Check sheet for the modelled part. Datum: model origin and axes. Units: mm. Face numbers are marked on the shaded views. Coordinates: 2 decimals unless noted, no trailing zeros. Loops run counter-clockwise (first coordinate to the right, second up) from the corner with the lowest first, then second, coordinate; pieces in that order, holes last. Notation, with made-up numbers: (78.5, -30) -> (85.5, -30) arc R16 ccw to (85.5, -26) -> close; hole circle Ø3 at (-26, -17). An arc over 180 degrees is marked (long way). Use CSV: the item, a comma, the result in double quotes. Start each with the question number.
1. Thickness scan on L1, parallel to Y at x = 52.1, z = -4.4; L2, parallel to Z at x = 45, y = 1.5; L3, parallel to X at y = 46, z = -2.9. Record the ranges inside material, lowest first.
2. Sectioned sample at B-B, the plane x = 47. Record the cut outline in (y, z).
3. Release check for a two-part mould opening along Y. For the marked faces 1 and 2 record: pulls with the +Y half, pulls with the -Y half, needs draft (parallel to the pull), parting line crosses it, or undercut.
4. Sectioned sample at A-A, the plane z = -0.7. Record the cut outline in (x, y), and give its area (3 significant figures).
5. Gauge pin test, flat ends, axial feed: pin 1 (3.5 mm diameter, centred on x = 52.1, y = 30.4, fed in from +Z); pin 2 (1 mm diameter, centred on x = 41, y = 32, fed in from +Z); pin 3 (2.5 mm diameter, centred on x = 0, y = 0, fed in from +Z). Record the tip position at first contact, or that the pin passes through.
6. Sectioned sample at C-C, the plane y = 23.5. Record the cut outline in (x, z), and give its area (3 significant figures).
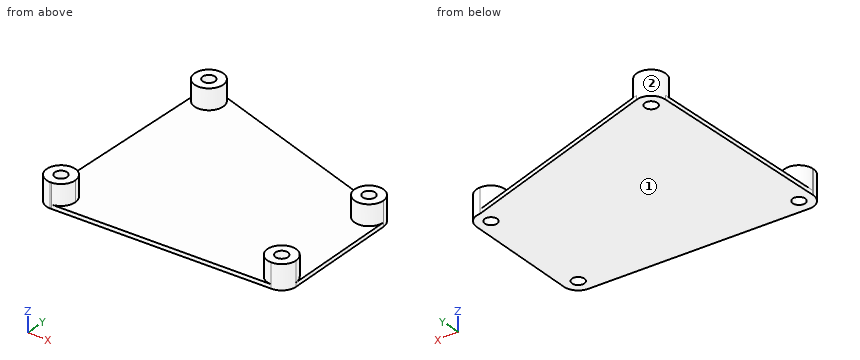
```python
from build123d import *

# Parameters (mm, degrees)
SKETCH1_R           = 3.5
SKETCH1_R_2         = 1.5
BOSS_EXTRUDE2_DEPTH = 6
CUT_EXTRUDE2_DEPTH  = 5


with BuildPart() as part:
    # Sketch1 → Boss-Extrude2 (new body)
    # profile 1 of 5: a face of its own
    with BuildSketch(Plane.XY):
        with BuildLine():
            ThreePointArc((4.8, 45.6), (1.3, 42.1), (-2.2, 45.6))
            Line((-2.2, 45.6), (-3.49431537, 0.199399342))
            ThreePointArc((-3.49431537, 0.199399342), (0.099740178, 3.498578554), (3.5, 0))
            ThreePointArc((3.5, 0), (2.590648868, -2.353409961), (0.33512089, -3.483919343))
            Line((0.33512089, -3.483919343), (52.1, -1))
            ThreePointArc((52.1, -1), (49.625126266, 4.974873734), (55.6, 2.5))
            Line((55.6, 2.5), (55.6, 30.4))
            ThreePointArc((55.6, 30.4), (49.625126266, 27.925126266), (52.1, 33.9))
            Line((52.1, 33.9), (2.312759359, 48.950271404))
            ThreePointArc((2.312759359, 48.950271404), (4.110218653, 47.686305616), (4.8, 45.6))
        make_face()
    # profile 2 of 5: a face of its own
    with BuildSketch(Plane.XY):
        with Locations((1.3, 45.6)):
            Circle(SKETCH1_R)
        with Locations((1.3, 45.6)):
            Circle(SKETCH1_R_2, mode=Mode.SUBTRACT)
    # profile 3 of 5: a face of its own
    with BuildSketch(Plane.XY):
        with Locations((52.1, 30.4)):
            Circle(SKETCH1_R)
        with Locations((52.1, 30.4)):
            Circle(SKETCH1_R_2, mode=Mode.SUBTRACT)
    # profile 4 of 5: a face of its own
    with BuildSketch(Plane.XY):
        with Locations((52.1, 2.5)):
            Circle(SKETCH1_R)
        with Locations((52.1, 2.5)):
            Circle(SKETCH1_R_2, mode=Mode.SUBTRACT)
    # profile 5 of 5: a face of its own
    with BuildSketch(Plane.XY):
        with BuildLine():
            ThreePointArc((3.5, 0), (0.099740178, 3.498578554), (-3.49431537, 0.199399342))
            Line((-3.49431537, 0.199399342), (-3.5, 0))
            ThreePointArc((-3.5, 0), (-2.474873734, -2.474873734), (0, -3.5))
            Line((0, -3.5), (0.33512089, -3.483919343))
            ThreePointArc((0.33512089, -3.483919343), (2.590648868, -2.353409961), (3.5, 0))
        make_face()
        Circle(SKETCH1_R_2, mode=Mode.SUBTRACT)
    extrude(amount=-BOSS_EXTRUDE2_DEPTH)

    # Sketch1<3> → Cut-Extrude2 (cut)
    with BuildSketch(Plane.XY):
        with BuildLine():
            ThreePointArc((4.8, 45.6), (1.3, 42.1), (-2.2, 45.6))
            Line((-2.2, 45.6), (-3.49431537, 0.199399342))
            ThreePointArc((-3.49431537, 0.199399342), (0.099740178, 3.498578554), (3.5, 0))
            ThreePointArc((3.5, 0), (2.590648868, -2.353409961), (0.33512089, -3.483919343))
            Line((0.33512089, -3.483919343), (52.1, -1))
            ThreePointArc((52.1, -1), (49.625126266, 4.974873734), (55.6, 2.5))
            Line((55.6, 2.5), (55.6, 30.4))
            ThreePointArc((55.6, 30.4), (49.625126266, 27.925126266), (52.1, 33.9))
            Line((52.1, 33.9), (2.312759359, 48.950271404))
            ThreePointArc((2.312759359, 48.950271404), (4.110218653, 47.686305616), (4.8, 45.6))
        make_face()
    extrude(amount=-CUT_EXTRUDE2_DEPTH, mode=Mode.SUBTRACT)


solid = part.part
```
Completed:
1,L1,"-1 to 1, 4 to 6, 26.9 to 28.9, 31.9 to 33.9"
1,L2,"-6 to -5"
1,L3,"-2.18 to -0.15, 2.75 to 4.78"
2,outline,"(-1.24, -6) -> (35.44, -6) -> (35.44, -5) -> (-1.24, -5) -> close"
3,face 1,"needs draft"
3,face 2,"undercut"
4,outline,"(-3.5, 0) arc R3.5 ccw to (0, -3.5) -> (0.34, -3.48) arc R3.5 ccw (long way) to (-3.49, 0.2) -> close; circle Ø7 at (1.3, 45.6); circle Ø7 at (52.1, 2.5); circle Ø7 at (52.1, 30.4); hole circle Ø3 at (0, 0); hole circle Ø3 at (1.3, 45.6); hole circle Ø3 at (52.1, 2.5); hole circle Ø3 at (52.1, 30.4)"
4,area,"126 mm²"
5,pin 1,"z = 0"
5,pin 2,"z = -5"
5,pin 3,"through"
6,outline,"(-2.83, -6) -> (55.6, -6) -> (55.6, -5) -> (-2.83, -5) -> close"
6,area,"58.4 mm²"
